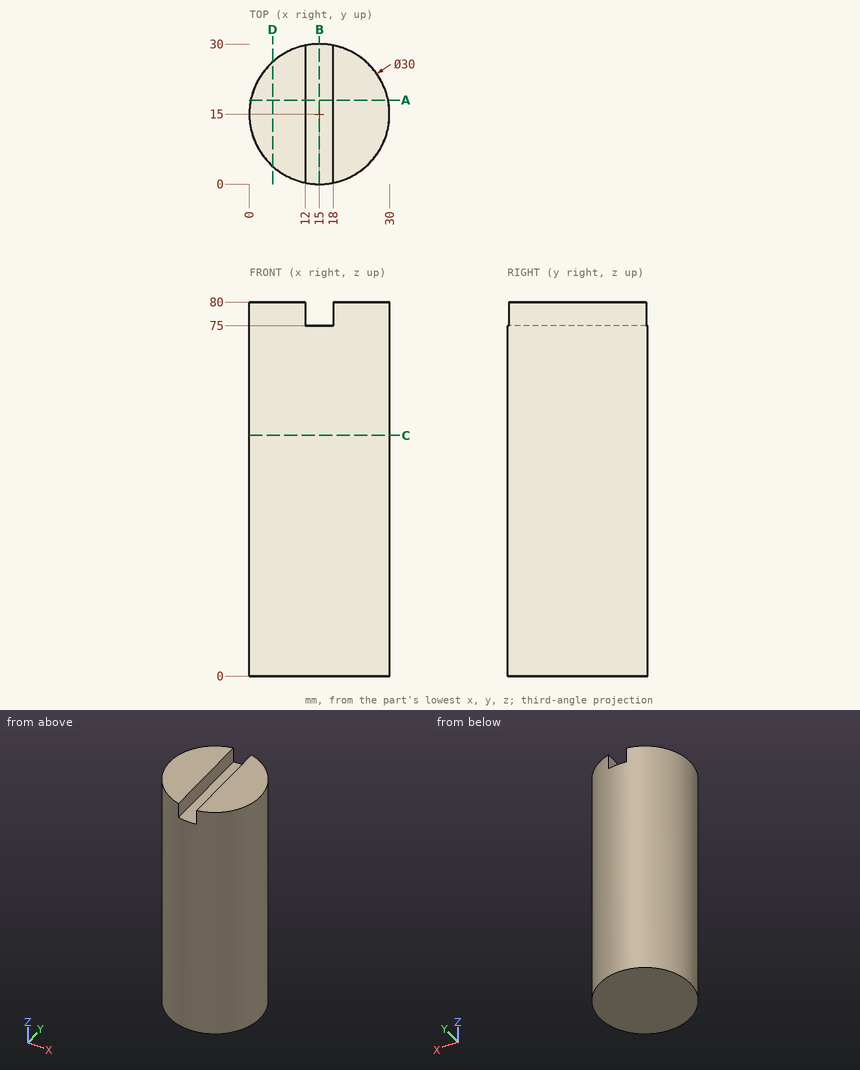
Geometry: see drawing. Coordinates: mm, zero at the bounding-box minimum. Give positions to 0.01 mm unless a question says otherwise; leave off trailing zeros. Write each loop counter-clockwise with the first axis right and the second up, starting at its lowest first coordinate (ties: lowest second). Pieces come first, ordered by that corner, then holes. Notation, with made-up numbers: (55.5, 46.25) -> (71.5, 46.25) arc R19 cw to (71.5, 54.25) -> close; hole circle Ø2 at (87.25, 66). An arc over 180 degrees is marked (long way). Use one line per item in the form item = value. Start each with the question number.
1) Section query A-A on y = 18. Return the cut outline in (x, z).
2) Section query C-C on z = 51.5. Return the cut outline in (x, y).
3) Section query D-D on x = 5. Return the cut outline in (y, z), then the cut area to 3 significant figures.
4) Pin query (flat end, axial travel): pin 1 (2 mm diameter, centred on y = 18, z = 34.5, fed in from +X); pin 2 (2 mm diameter, centred on x = 17.5, z = 57.5, fed in from -Y); pin 3 (1.5 mm diameter, centred on y = 9.5, z = 77.5, fed in from +X). Return the tip coordinate at first contact, or that it passes through.
5) Section query B-B on x = 15. Return the cut outline in (y, z).
6) Ray query, probe 1 along X at (y, z) = (18, 24); probe 2 along Z at (x, y) = (15, 17); probe 3 along X at (y, z) = (9.5, 75.5). Return the intervals inside material, ascending. Write a range as from..to.
Outcome:
q1.outline = (0.3, 0) -> (29.7, 0) -> (29.7, 80) -> (18, 80) -> (18, 75) -> (12, 75) -> (12, 80) -> (0.3, 80) -> close
q2.outline = circle Ø30 at (15, 15)
q3.outline = (3.82, 0) -> (26.18, 0) -> (26.18, 80) -> (3.82, 80) -> close
q3.area = 1,790 mm^2
q4.pin_1 = 29.87
q4.pin_2 = 0.08
q4.pin_3 = 29.23
q5.outline = (0, 0) -> (30, 0) -> (30, 75) -> (0, 75) -> close
q6.probe_1 = 0.3..29.7
q6.probe_2 = 0..75
q6.probe_3 = 1.04..12, 18..28.96
